from build123d import *

# Parameters (mm, degrees)
SKETCH1_W          = 889
SKETCH1_H          = 31.75
EXTRUDE1_DEPTH     = 28.575
EXTRUDE2_REACH     = 891
SKETCH2_W          = 25.4
SKETCH2_H          = 25.4
HOLE1_D            = 6.35
HOLE1_DEPTH        = 3.175
LPATTERN1_COUNT    = 35
LPATTERN1_PITCH    = 25.4
HOLE2_D            = 9.652
HOLE2_DEPTH        = 3.175
LPATTERN2_COUNT    = 12
LPATTERN2_PITCH    = 25.4
HOLE3_D            = 9.652
HOLE3_DEPTH        = 3.175
HOLE4_D            = 9.652
HOLE4_DEPTH        = 3.175
LPATTERN3_COUNT    = 12
LPATTERN3_PITCH    = 25.4
HOLE5_D            = 3.175
HOLE5_DEPTH        = 3.175
HOLE6_D            = 6.35
HOLE6_DEPTH        = 3.175
LPATTERN4_COUNT    = 35
LPATTERN4_PITCH    = 25.4
FILLET1_R          = 3.175
FILLET2_R          = 3.175
FILLET3_R          = 6.35
FILLET4_R          = 6.35
SKETCH16_W         = 145.760071232
SKETCH16_H         = 71.504803879
CUT_EXTRUDE2_DEPTH = 75


with BuildPart() as part:
    # Sketch1 → Extrude1 (new body)
    with BuildSketch(Plane.XY.offset(3.175)):
        with Locations((428.480011997, 8.672957166)):
            Rectangle(SKETCH1_W, SKETCH1_H)
    extrude(amount=-EXTRUDE1_DEPTH)

    # Sketch2 → Extrude2 (cut, up to next)
    with BuildSketch(Plane.ZY.offset(16.019988003), mode=Mode.PRIVATE) as extrude2_sk1:
        with Locations((-12.7, 8.672957166)):
            Rectangle(SKETCH2_W, SKETCH2_H)
    extrude2_tool1 = extrude(extrude2_sk1.sketch, amount=-EXTRUDE2_REACH, mode=Mode.PRIVATE) & part.part
    add(extrude2_tool1.solids().sort_by_distance((-16.019988, 8.672957, -12.7))[0], mode=Mode.SUBTRACT)

    # Hole1
    with Locations(Plane(origin=(0, 24.547957166, 0), x_dir=(-1, 0, 0), z_dir=(0, 1, 0))):
        with Locations((3.319988003, -12.7)):
            hole1 = Hole(HOLE1_D / 2, depth=HOLE1_DEPTH)

    # LPattern1: Hole1 ×35
    with Locations(*[(i * LPATTERN1_PITCH, 0, 0) for i in range(1, LPATTERN1_COUNT)]):
        add(hole1, mode=Mode.SUBTRACT)

    # Hole2
    with Locations(Plane.XY.offset(3.175)):
        with Locations((66.530011997, 10.577957166)):
            hole2 = Hole(HOLE2_D / 2, depth=HOLE2_DEPTH)

    # LPattern2: Hole2 ×12, 8 skipped
    with Locations(*[(i * LPATTERN2_PITCH, 0, 0) for i in range(1, LPATTERN2_COUNT) if i not in (2, 3, 4, 5, 6, 7, 8, 9)]):
        add(hole2, mode=Mode.SUBTRACT)

    # Hole3
    with Locations(Plane.XY.offset(3.175)):
        with Locations((428.480011997, 6.767957166)):
            Hole(HOLE3_D / 2, depth=HOLE3_DEPTH)

    # Hole4
    with Locations(Plane.XY.offset(3.175)):
        with Locations((511.030011997, 10.577957166)):
            hole4 = Hole(HOLE4_D / 2, depth=HOLE4_DEPTH)

    # LPattern3: Hole4 ×12, 8 skipped
    with Locations(*[(i * LPATTERN3_PITCH, 0, 0) for i in range(1, LPATTERN3_COUNT) if i not in (2, 3, 4, 5, 6, 7, 8, 9)]):
        add(hole4, mode=Mode.SUBTRACT)

    # Hole5
    with Locations(Plane.XY.offset(3.175)):
        with Locations((669.780011997, 8.672957166)):
            Hole(HOLE5_D / 2, depth=HOLE5_DEPTH)

    # Hole6
    with Locations(Plane(origin=(0, -4.027042834, 0), x_dir=(-1, 0, 0), z_dir=(0, 1, 0))):
        with Locations((3.319988003, -12.7)):
            hole6 = Hole(HOLE6_D / 2, depth=HOLE6_DEPTH)

    # LPattern4: Hole6 ×35
    with Locations(*[(i * LPATTERN4_PITCH, 0, 0) for i in range(1, LPATTERN4_COUNT)]):
        add(hole6, mode=Mode.SUBTRACT)

    # Fillet1
    fillet1_edges = [part.edges().sort_by_distance(p)[0] for p in [
        (428.480011997, 21.372957166, 0),
    ]]
    fillet(fillet1_edges, radius=FILLET1_R)

    # Fillet2
    fillet2_edges = [part.edges().sort_by_distance(p)[0] for p in [
        (428.480011997, -4.027042834, 0),
    ]]
    fillet(fillet2_edges, radius=FILLET2_R)

    # Fillet3
    fillet3_edges = [part.edges().sort_by_distance(p)[0] for p in [
        (428.480011997, -7.202042834, 3.175),
    ]]
    fillet(fillet3_edges, radius=FILLET3_R)

    # Fillet4
    fillet4_edges = [part.edges().sort_by_distance(p)[0] for p in [
        (428.480011997, 24.547957166, 3.175),
    ]]
    fillet(fillet4_edges, radius=FILLET4_R)

    # Sketch16 → Cut-Extrude2 (cut)
    with BuildSketch(Plane(origin=(0, 24.547957166, 0), x_dir=(1, 0, 0), z_dir=(0, 1, 0))):
        with Locations((40.099976381, -10.352401939)):
            Rectangle(SKETCH16_W, SKETCH16_H)
    extrude(amount=-CUT_EXTRUDE2_DEPTH, mode=Mode.SUBTRACT)


solid = part.part
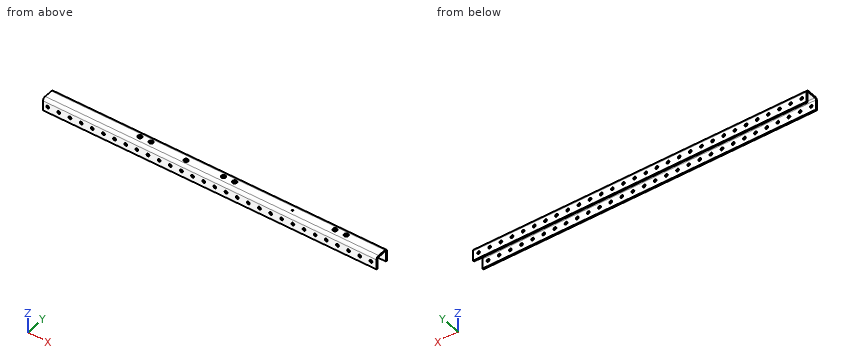
The listing builds one solid part. Answer for the finished solid, in the listing's coordinates (mm). Give positions to 0.01 mm unless a question says otherwise; leave off trailing zeros. Order: outer loops, then holes, each group sorted by start corner. A loop starts at its lowest first (then second) coordinate and runs counter-clockwise, first axis right, second up. Notation, with made-up numbers: (74.25, 12) -> (111.25, 12) arc R29 ccw to (111.25, 44) -> close; hole circle Ø3 at (49.5, 49). An arc over 180 degrees is marked (long way). Put each result on its own line as item: value.
Item 1: A cutting plane is placed at B-B on x = 644. Give the vertices of the cut face in (y, z) (3 decimals).
Established:
outline: (-7.202, -25.4) -> (-4.027, -25.4) -> (-4.027, -3.175) arc R3.175 cw to (-0.852, 0) -> (18.198, 0) arc R3.175 cw to (21.373, -3.175) -> (21.373, -25.4) -> (24.548, -25.4) -> (24.548, -3.175) arc R6.35 ccw to (18.198, 3.175) -> (-0.852, 3.175) arc R6.35 ccw to (-7.202, -3.175) -> close
Item 2: Given P1, Ø2, axis at y = -2, z = -22, coming from the -X side; P2, Ø5, axis at x = 571.5, y = 5, coming from the -Z side, each flat-ended and moving along its own axis, determine where each tip first touches the part or whether it passes through.
Established:
P1: passes through
P2: stops at z = 0
Item 3: A cutting plane is placed at A-A on z = -21. Give the vertices of the cut face in (x, y).
Established:
outline: (112.98, -7.2) -> (872.98, -7.2) -> (872.98, -4.03) -> (112.98, -4.03) -> close; (112.98, 21.37) -> (872.98, 21.37) -> (872.98, 24.55) -> (112.98, 24.55) -> close
Item 4: Straight lines are drawn through the part: line 1 (Y direction, x = 245, z = -13); line 2 (Y direction, x = 547, z = -2.75); line 3 (Z direction, x = 376.5, y = 5.5) (3 decimals). For each, find the intervals that lie inside material, in ascending order.
Established:
line 1: y = -7.2 to -4.03, 21.37 to 24.55
line 2: y = -7.19 to -4, 21.34 to 24.53
line 3: z = 0 to 3.175
